Geometry: final body of the model. Coordinates: model frame, mm. Face numbers are marked on the shaded views. Give positions to 0.01 mm unless a question says otherwise; leave off trailing zeros. Write each loop counter-clockwise with the first axis right and the second up, starting at its lowest first coordinate (ties: lowest second). Pieces come first, ordered by that corner, then holes. Notation, with made-up numbers: (70.25, 72) -> (89.25, 72) arc R11 ccw to (89.25, 78) -> close; hole circle Ø5 at (2.5, 77). An arc over 180 degrees is marked (long way). Answer as a JSON object with one key per item and string values.
from build123d import *

# Parameters (mm, degrees)
SKETCH_1_W          = 36
SKETCH_1_H          = 8
SKETCH_1_R          = 2
EXTRUDE_1_DEPTH     = 39
SKETCH_3_R          = 9
CUT_EXTRUDE_1_DEPTH = 10


with BuildPart() as part:
    # 草图1 → 凸台-拉伸1 (new body)
    with BuildSketch(Plane(origin=(0, 0, 0), x_dir=(1, 0, 0), z_dir=(0, 1, 0))):
        Rectangle(SKETCH_1_W, SKETCH_1_H)
        with Locations(Location((12.5, 0, 0), (0, 0, 270))):
            Circle(SKETCH_1_R, mode=Mode.SUBTRACT)
        with Locations(Location((-12.5, 0, 0), (0, 0, 90))):
            Circle(SKETCH_1_R, mode=Mode.SUBTRACT)
    extrude(amount=EXTRUDE_1_DEPTH)

    # 草图3 → 切除-拉伸1 (cut)
    with BuildSketch(Plane.XY.offset(4)):
        with Locations((0, 23.5)):
            Circle(SKETCH_3_R)
    extrude(amount=-CUT_EXTRUDE_1_DEPTH, mode=Mode.SUBTRACT)


solid = part.part
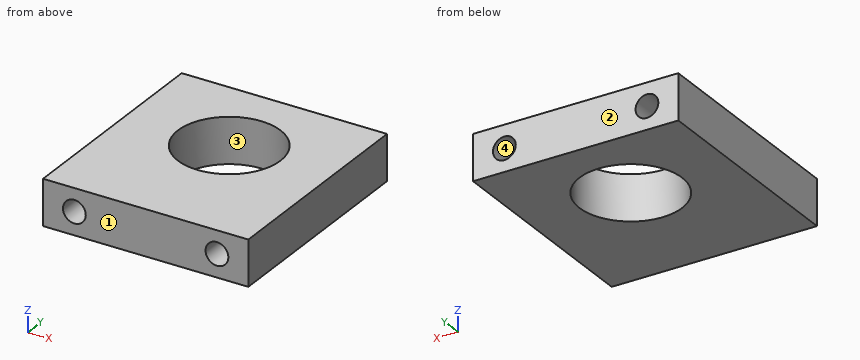
Q1. Cut plane D-D (y = 36). Return the cut outline in (x, z).
Values:
{"outline": "(-18, -4) -> (18, -4) -> (18, 4) -> (-18, 4) -> close; hole circle Ø4 at (-12.5, 0); hole circle Ø4 at (12.5, 0)"}
Q2. Cut plane C-C (y = 20.5). Return the cut outline in (x, z).
Values:
{"outline": "(-18, -4) -> (-8.49, -4) -> (-8.49, 4) -> (-18, 4) -> close; (8.49, -4) -> (18, -4) -> (18, 4) -> (8.49, 4) -> close; hole circle Ø4 at (-12.5, 0); hole circle Ø4 at (12.5, 0)"}
Q3. Material intervals for L1, parallel to X at y = 26, z = 0; L2, parallel to X at y = 20, z = 0; L3, parallel to X at y = 12, z = 0.5, sorted ascending. Write a range as from..to.
Values:
{"L1": "-18..-14.5, -10.5..-8.65, 8.65..10.5, 14.5..18", "L2": "-18..-14.5, -10.5..-8.29, 8.29..10.5, 14.5..18", "L3": "-18..-14.44, -10.56..10.56, 14.44..18"}
Q4. Mould query, pull axis Y, two halves, no side actions, for the marked faces 1, 2, 3 and 4. Classes: pulls with the +Y half, pulls with the -Y half, needs draft (parallel to the pull), parting line crosses it, or undercut.
Values:
{"face 1": "pulls with the -Y half", "face 2": "pulls with the +Y half", "face 3": "undercut", "face 4": "needs draft"}
Q5. Cut plane B-B (x = -12.5). Return the cut outline in (y, z), and give its area (3 significant figures).
Values:
{"outline": "(0, -4) -> (39, -4) -> (39, -2) -> (0, -2) -> close; (0, 2) -> (39, 2) -> (39, 4) -> (0, 4) -> close", "area": "156 mm²"}
Q6. First-contact query: P1, Ø1, axis at x = -12, z = -1, coming from the +Y side. Flat tip, straight axial feed; report the tip coordinate or a pass-through.
Values:
{"P1": "through"}
Q7. Cut plane A-A (z = 0). Return the cut outline in (x, y).
Values:
{"outline": "(-18, 0) -> (-14.5, 0) -> (-14.5, 39) -> (-18, 39) -> close; (-10.5, 0) -> (10.5, 0) -> (10.5, 39) -> (-10.5, 39) -> close; (14.5, 0) -> (18, 0) -> (18, 39) -> (14.5, 39) -> close; hole circle Ø18 at (0, 23.5)"}
